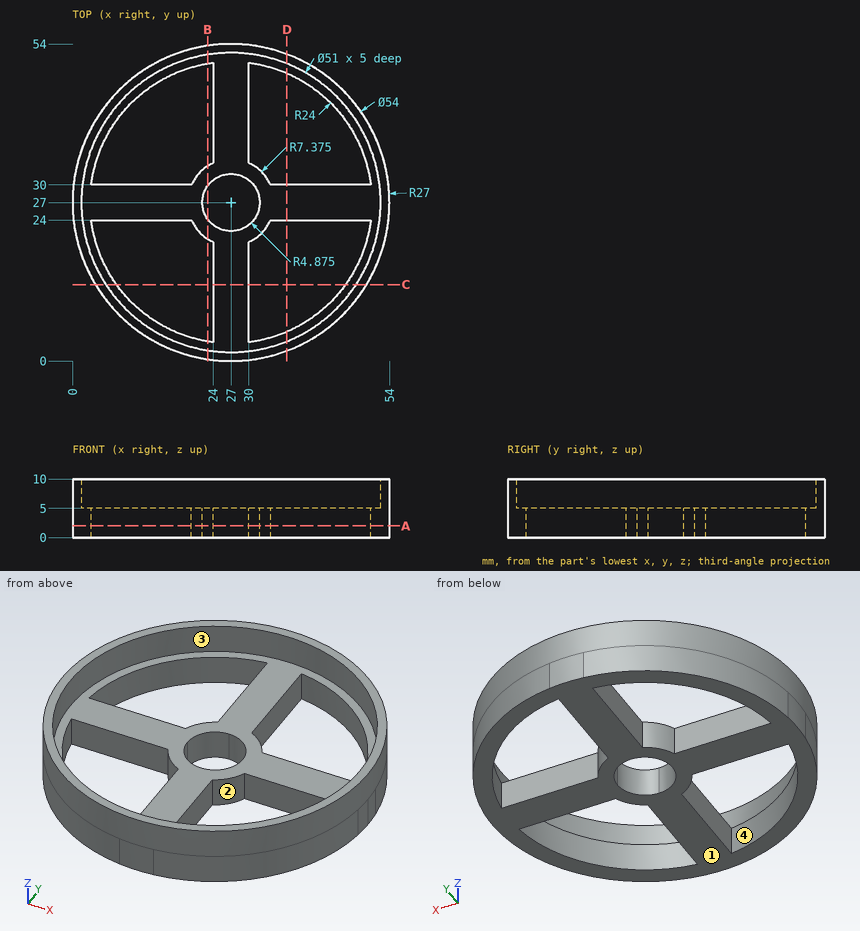
Design review of the part shown in the three views and the two pictorial views. Dimensions are in mm from the part's minimum x, y and z. A direction names the side the tool comes from. Round coordinates to 2 decimals unless told otherwise and drop trailing zeros. Write each loop counter-clockwise with the first axis right and the second up, starting at its lowest first coordinate (ties: lowest second). Pieces come first, ordered by that corner, then holes. Notation, with made-up numbers: (50.25, 85) - (64.25, 85) arc R15 ccw to (64.25, 113) - close; hole circle Ø5 at (78.25, 69). An arc over 180 degrees is marked (long way). Answer as CSV lines item,"result". Start each with the question number.
(1) Add section B-B, the plane x = 23. State the section outline as (y, z) points.
(2) For pin 1 (1.5 mm diameter, centred on y = 41, z = 2, fed in from -X); pin 2 (2.5 mm diameter, centred on y = 16, z = 1.5, fed in from -X); pin 3 (3 mm diameter, centred on y = 31.5, z = 3.5, fed in from +X); pin 4 (8 mm diameter, centred on x = 46, y = 40, fed in from +Z), all flat-tipped, find the tip position at first contact; note any pin that passes through.
(3) Add section C-C, the plane y = 13. State the section outline as (x, z) points.
(4) Machinability: for the marked faces 3 and 4, which of the approach directions +Z, -Z, +X, -X, +Y, -Y give a long, thin tool a straight path to every point of the face, cutting with its end or side? Answer none if there is none.
(5) Mouldability with a two-part tool opening along X and no side actions: class the marked faces 1 and 2 as +X half, -X half, draft (parallel to the pull), parting line (faces both ways), or undercut.
(6) Add section A-A, the plane z = 2. State the section outline as (x, y) points (3 decimals), plus the area to 3 significant figures.
(7) For line 1 (X direction, y = 36.5, z = 3.5); line 2 (X direction, y = 7, z = 4.5); line 3 (Y direction, x = 27, z = 6.05), list the stretches that pass through material, from the lowest coordinate up.
(8) Add section D-D, the plane x = 36.5. State the section outline as (y, z) points.
From the geometry:
1,outline,"(0.3, 0) - (3.34, 0) - (3.34, 5) - (1.82, 5) - (1.82, 10) - (0.3, 10) - close; (20.8, 0) - (24.21, 0) - (24.21, 5) - (20.8, 5) - close; (29.79, 0) - (33.2, 0) - (33.2, 5) - (29.79, 5) - close; (50.66, 0) - (53.7, 0) - (53.7, 10) - (52.18, 10) - (52.18, 5) - (50.66, 5) - close"
2,pin 1,"stops at x = 3.47"
2,pin 2,"stops at x = 1.82"
2,pin 3,"stops at x = 53.83"
2,pin 4,"stops at z = 10"
3,outline,"(3.91, 0) - (7.51, 0) - (7.51, 5) - (5.69, 5) - (5.69, 10) - (3.91, 10) - close; (24, 0) - (30, 0) - (30, 5) - (24, 5) - close; (46.49, 0) - (50.09, 0) - (50.09, 10) - (48.31, 10) - (48.31, 5) - (46.49, 5) - close"
4,face 3,"+Z"
4,face 4,"+Z, -Z"
5,face 1,"draft"
5,face 2,"undercut"
6,outline,"circle Ø54 at (27, 27); hole (3.188, 24) arc R24 ccw to (24, 3.188) - (24, 20.263) arc R7.375 cw to (20.263, 24) - close; hole (3.188, 30) - (20.263, 30) arc R7.375 cw to (24, 33.737) - (24, 50.812) arc R24 ccw to start; hole circle Ø9.75 at (27, 27); hole (30, 3.188) arc R24 ccw to (50.812, 24) - (33.737, 24) arc R7.375 cw to (30, 20.263) - close; hole (30, 33.737) arc R7.375 cw to (33.737, 30) - (50.812, 30) arc R24 ccw to (30, 50.812) - close"
6,area,"979 mm²"
7,line 1,"x = 1.73 to 4.96, 24 to 30, 49.04 to 52.27"
7,line 2,"x = 8.86 to 13.73, 24 to 30, 40.27 to 45.14"
7,line 3,"y = 0 to 1.5, 52.5 to 54"
8,outline,"(1.73, 0) - (4.96, 0) - (4.96, 5) - (3.34, 5) - (3.34, 10) - (1.73, 10) - close; (24, 0) - (30, 0) - (30, 5) - (24, 5) - close; (49.04, 0) - (52.27, 0) - (52.27, 10) - (50.66, 10) - (50.66, 5) - (49.04, 5) - close"
